Here's how the part is built. I have some questions about the finished solid (model axes, mm). Coordinates: 2 decimals unless noted, no trailing zeros. Write each loop counter-clockwise with the first axis right and the second up, starting at its lowest first coordinate (ties: lowest second). Pieces come first, ordered by that corner, then holes.
Item 1: I'm going to push flat-ended pins straight in: P1, Ø2, axis at y = -2, z = -33.5, coming from the +X side; P2, Ø3, axis at y = -1.5, z = -63, coming from the +X side; P3, Ø3, axis at y = -0.5, z = -46, coming from the +X side. Where does each tip first touch, or does it pass through?
Item 2: I want a section at A-A (z = -50.8). Please give me the cut outline in (x, y) (3 decimals).
Item 3: Please list where these lines run through material, in increasing order: line 1 (X direction, y = 1.25, z = -63.5); line 2 (Z direction, x = 26, y = -2.75); line 3 (X direction, y = -2, z = -65.5).
Item 4: I want a section at C-C (x = 38.1). Please give me the cut outline in (y, z) (3 decimals).
Item 5: I want a section at D-D (z = 6). Please give me the cut outline in (x, y) (3 decimals), and give its area (3 significant figures).
Item 6: I want a section at B-B (y = 1.75). Count the separate pieces of the cut face and the enclosed holes in it, and give its area (3 significant figures).
from build123d import *
from build123d.topology import SkipClean

# Parameters (mm, degrees)
SKETCH1_R           = 2.5527
BOSS_EXTRUDE1_DEPTH = 3.175


with BuildPart() as part:
    # Sketch1 → Boss-Extrude1 (new, symmetric)
    # profile 1 of 4: a face of its own
    with SkipClean():  # the faces are left unmerged after this step: merging them gives an invalid solid
        with BuildSketch(Plane(origin=(0, 0, 0), x_dir=(1, 0, 0), z_dir=(0, 1, 0))):
            with BuildLine():
                Line((-12.7, 63.5), (-12.7, 0))
                ThreePointArc((-12.7, 0), (-9.837305348, 8.032273868), (-2.539775829, 12.44345365))
                ThreePointArc((-2.539775829, 12.44345365), (-0.128435844, 15.24946691), (2.5527, 12.7))
                Line((2.5527, 12.7), (12.7, 12.7))
                Line((12.7, 12.7), (12.7, 63.5))
                ThreePointArc((12.7, 63.5), (0, 76.2), (-12.7, 63.5))
            make_face()
            with Locations(Location((0, 25.4, 0), (0, 0, 270))):
                Circle(SKETCH1_R, mode=Mode.SUBTRACT)
            with Locations(Location((0, 38.1, 0), (0, 0, 270))):
                Circle(SKETCH1_R, mode=Mode.SUBTRACT)
            with Locations(Location((0, 50.8, 0), (0, 0, 270))):
                Circle(SKETCH1_R, mode=Mode.SUBTRACT)
            with Locations(Location((0, 63.5, 0), (0, 0, 270))):
                Circle(SKETCH1_R, mode=Mode.SUBTRACT)
        # profile 2 of 4: a face of its own
        with BuildSketch(Plane(origin=(0, 0, 0), x_dir=(1, 0, 0), z_dir=(0, 1, 0))):
            with BuildLine():
                Line((12.7, 12.7), (63.5, 12.7))
                ThreePointArc((63.5, 12.7), (27.578975516, 27.578975516), (12.7, 63.5))
                Line((12.7, 63.5), (12.7, 12.7))
            make_face()
        # profile 3 of 4: a face of its own
        with BuildSketch(Plane(origin=(0, 0, 0), x_dir=(1, 0, 0), z_dir=(0, 1, 0))):
            with BuildLine():
                Line((0, -12.7), (63.5, -12.7))
                ThreePointArc((63.5, -12.7), (76.2, 0), (63.5, 12.7))
                Line((63.5, 12.7), (12.7, 12.7))
                Line((12.7, 12.7), (12.7, 2.5527))
                ThreePointArc((12.7, 2.5527), (14.50503148, 1.80503148), (15.2527, 0))
                ThreePointArc((15.2527, 0), (14.411927484, -1.893563196), (12.44345365, -2.539775829))
                ThreePointArc((12.44345365, -2.539775829), (8.032273868, -9.837305348), (0, -12.7))
            make_face()
            with Locations(Location((25.4, 0, 0), (0, 0, 270))):
                Circle(SKETCH1_R, mode=Mode.SUBTRACT)
            with Locations(Location((38.1, 0, 0), (0, 0, 270))):
                Circle(SKETCH1_R, mode=Mode.SUBTRACT)
            with Locations(Location((50.8, 0, 0), (0, 0, 270))):
                Circle(SKETCH1_R, mode=Mode.SUBTRACT)
            with Locations(Location((63.5, 0, 0), (0, 0, 270))):
                Circle(SKETCH1_R, mode=Mode.SUBTRACT)
        # profile 4 of 4: a face of its own
        with BuildSketch(Plane(origin=(0, 0, 0), x_dir=(1, 0, 0), z_dir=(0, 1, 0))):
            with BuildLine():
                ThreePointArc((-12.7, 0), (-8.980256121, -8.980256121), (0, -12.7))
                ThreePointArc((0, -12.7), (8.032273868, -9.837305348), (12.44345365, -2.539775829))
                ThreePointArc((12.44345365, -2.539775829), (10.15053309, 0.128435844), (12.7, 2.5527))
                Line((12.7, 2.5527), (12.7, 12.7))
                Line((12.7, 12.7), (2.5527, 12.7))
                ThreePointArc((2.5527, 12.7), (0.128435844, 10.15053309), (-2.539775829, 12.44345365))
                ThreePointArc((-2.539775829, 12.44345365), (-9.837305348, 8.032273868), (-12.7, 0))
            make_face()
            with Locations(Location((0, 0, 0), (0, 0, 270))):
                Circle(SKETCH1_R, mode=Mode.SUBTRACT)
        extrude(amount=BOSS_EXTRUDE1_DEPTH, both=True)


solid = part.part
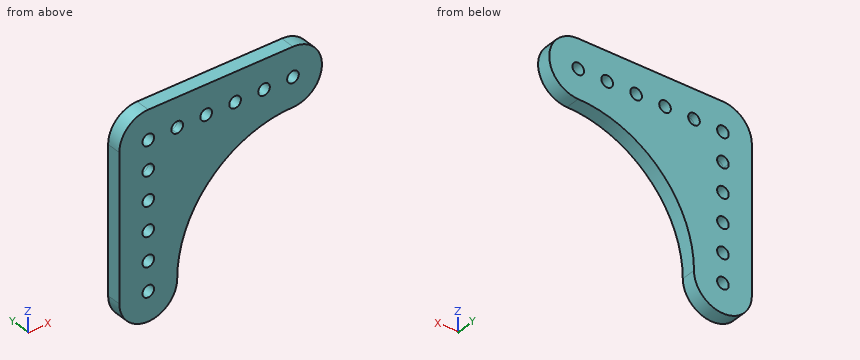
Answer:
1. P1: stops at x = 23.26
1. P2: stops at x = 12.74
1. P3: stops at x = 16.39
2. outline: (-12.7, -3.175) - (-2.553, -3.175) - (-2.553, 3.175) - (-12.7, 3.175) - close; (2.553, -3.175) - (14.313, -3.175) - (14.313, 3.175) - (2.553, 3.175) - close
3. line 1: x = -12.7 to -2.55, 2.55 to 12.7
3. line 2: z = -29.23 to -2.48, 2.48 to 12.7
3. line 3: x = -12.54 to -1.59, 1.59 to 12.54
4. outline: (-3.175, -19.506) - (3.175, -19.506) - (3.175, -2.553) - (-3.175, -2.553) - close; (-3.175, 2.553) - (3.175, 2.553) - (3.175, 12.7) - (-3.175, 12.7) - close
5. outline: (-11.193, -3.175) - (74.693, -3.175) - (74.693, 3.175) - (-11.193, 3.175) - close
5. area: 545 mm2
6. separate pieces: 1
6. enclosed holes: 11
6. area: 4,030 mm2
